Geometry: final body of the model. Coordinates: model frame, mm. A direction names the side the tool comes from. Round coordinates to 2 decimals unless told otherwise and drop trailing zeros. Write each loop counter-clockwise with the first axis right and the second up, starting at its lowest first coordinate (ties: lowest second). Pieces come first, ordered by that corner, then holes. Notation, with made-up numbers: (9, 48.25) -> (32, 48.25) arc R19 ccw to (32, 75.25) -> close; hole circle Ø7 at (2, -26). An arc over 180 degrees is marked (long way). Use one line per item in the form item = value. Start each with the question number.
1. Cut plane C-C, the plane y = 11. Return the cut outline in (x, z), plus the area to 3 significant figures.
2. Cut plane B-B, the plane z = 15. Return the cut outline in (x, y), plus the area to 3 significant figures.
3. Line query: L1, parallel to Z at x = 30, y = 9; L2, parallel to X at y = 2.5, z = 3.5; L3, parallel to Y at x = 18, z = 15. Output: solid intervals per line, ascending.
4. Cut plane D-D, the plane z = 11.5. Return the cut outline in (x, y).
5. Draft query along X for faces 1 (the face through (28, 7, 12.5)), 2 (the face through (19, 16, 9)), 3 (the face through (28, 14, 9)), 4 (the face through (28, 7, 5.5)). Return one class per face: pulls with the +X half, pulls with the -X half, needs draft (parallel to the pull), parting line crosses it, or undercut.
6. Pin query (flat end, axial travel): pin 1 Ø10.5 at (x, z) = (28, 5) entering from +Y. Return the tip coordinate at first contact, or that it passes through.
7. Cut plane A-A, the plane x = 29. Return the cut outline in (y, z).
8. Reachability of faces 5 (the face through (17, 9, 18)), 6 (the face through (28, 7, 16.5)) from +Z, -Z, +X, -X, +Y, -Y: full face, straight path, thin tool, end or side. Return the list, or none.
```python
from build123d import *

# Parameters (mm, degrees)
F1_DEPTH = 18
F3_DEPTH = 15


with BuildPart() as f1:
    # F0 (on Top) → F1 (new body)
    with BuildSketch(Plane.XY):
        Polygon((0, 18), (0, 0), (34, 0), (34, 14), (21, 14), (17, 18), align=None)
    extrude(amount=F1_DEPTH)

    # F2 (on Front) → F3 (cut)
    with BuildSketch(Plane.XZ):
        with BuildLine():
            ThreePointArc((33, 14.5), (32.414214, 15.914214), (31, 16.5))
            Line((31, 16.5), (25, 16.5))
            ThreePointArc((25, 16.5), (23.585786, 15.914214), (23, 14.5))
            ThreePointArc((23, 14.5), (23.585786, 13.085786), (25, 12.5))
            Line((25, 12.5), (31, 12.5))
            ThreePointArc((31, 12.5), (32.414214, 13.085786), (33, 14.5))
        make_face()
        with BuildLine():
            ThreePointArc((23, 3.5), (23.585786, 2.085786), (25, 1.5))
            Line((25, 1.5), (31, 1.5))
            ThreePointArc((31, 1.5), (32.414214, 2.085786), (33, 3.5))
            ThreePointArc((33, 3.5), (32.414214, 4.914214), (31, 5.5))
            Line((31, 5.5), (25, 5.5))
            ThreePointArc((25, 5.5), (23.585786, 4.914214), (23, 3.5))
        make_face()
    extrude(amount=-F3_DEPTH, mode=Mode.SUBTRACT)


solid = f1.part
```
Outcome:
q1.outline = (0, 0) -> (34, 0) -> (34, 18) -> (0, 18) -> close; hole (23, 3.5) arc R2 ccw to (25, 1.5) -> (31, 1.5) arc R2 ccw to (33, 3.5) arc R2 ccw to (31, 5.5) -> (25, 5.5) arc R2 ccw to start; hole (23, 14.5) arc R2 ccw to (25, 12.5) -> (31, 12.5) arc R2 ccw to (33, 14.5) arc R2 ccw to (31, 16.5) -> (25, 16.5) arc R2 ccw to start
q1.area = 539 mm^2
q2.outline = (0, 0) -> (23.06, 0) -> (23.06, 14) -> (21, 14) -> (17, 18) -> (0, 18) -> close; (32.94, 0) -> (34, 0) -> (34, 14) -> (32.94, 14) -> close
q2.area = 414 mm^2
q3.L1 = 0 to 1.5, 5.5 to 12.5, 16.5 to 18
q3.L2 = 0 to 23, 33 to 34
q3.L3 = 0 to 17
q4.outline = (0, 0) -> (34, 0) -> (34, 14) -> (21, 14) -> (17, 18) -> (0, 18) -> close
q5.face_1 = undercut
q5.face_2 = pulls with the +X half
q5.face_3 = needs draft
q5.face_4 = undercut
q6.pin_1 = 14
q7.outline = (0, 0) -> (14, 0) -> (14, 1.5) -> (0, 1.5) -> close; (0, 5.5) -> (14, 5.5) -> (14, 12.5) -> (0, 12.5) -> close; (0, 16.5) -> (14, 16.5) -> (14, 18) -> (0, 18) -> close
q8.face_5 = +Z, +X, -X, +Y, -Y
q8.face_6 = +Y, -Y
